Geometry check sheet. Reference: the model listing, model coordinates, mm. A direction names the side the tool comes from. Round coordinates to 2 decimals unless told otherwise and drop trailing zeros. Write each loop counter-clockwise with the first axis right and the second up, starting at its lowest first coordinate (ties: lowest second). Pieces come first, ordered by that corner, then holes. Notation, with made-up numbers: (-10, 74.5) - (22, 74.5) arc R11 cw to (22, 92.5) - close; hole circle Ø11 at (31.5, 13). An arc over 180 degrees is marked (long way). Return JSON: item names as keys, results as strings.
```python
from build123d import *

# Parameters (mm, degrees)
SKETCH_1_R      = 3.9
EXTRUDE_1_DEPTH = 20
SKETCH_2_R      = 5.636785761
SKETCH_2_R_2    = 2.651196968
EXTRUDE_2_DEPTH = 20


with BuildPart() as part:
    # 스케치1 → 보스-돌출1 (new body)
    with BuildSketch(Plane.XY):
        Circle(SKETCH_1_R)
    extrude(amount=EXTRUDE_1_DEPTH)

    # 스케치2 → 보스-돌출2 (add)
    with BuildSketch(Plane.XY):
        Circle(SKETCH_2_R)
        Circle(SKETCH_2_R_2, mode=Mode.SUBTRACT)
    extrude(amount=-EXTRUDE_2_DEPTH)


solid = part.part
```
(1) Section check D-D, the plane y = 3. Enter the section's corners in (x, z), plus the area to 3 significant figures.
Response values:
{"outline": "(-4.77, -20) - (4.77, -20) - (4.77, 0) - (2.49, 0) - (2.49, 20) - (-2.49, 20) - (-2.49, 0) - (-4.77, 0) - close", "area": "291 mm^2"}
(2) Material ranges on line 1 along Y through (x, z) = (0, -9.25); line 2 along Z through (x, y) = (-4, -3.5); line 3 along Z through (x, y) = (1.5, 2), recorded low to high. Write a range as [from, to].
Response values:
{"line 1": "y = [-5.64, -2.65], [2.65, 5.64]", "line 2": "z = [-20, 0]", "line 3": "z = [0, 20]"}
(3) Section check B-B, the plane z = -2. Enter the section's corners in (x, y).
Response values:
{"outline": "circle Ø11.27 at (0, 0); hole circle Ø5.3 at (0, 0)"}
(4) Section check A-A, the plane x = 0. Enter the section's corners in (y, z).
Response values:
{"outline": "(-5.64, -20) - (-2.65, -20) - (-2.65, 0) - (2.65, 0) - (2.65, -20) - (5.64, -20) - (5.64, 0) - (3.9, 0) - (3.9, 20) - (-3.9, 20) - (-3.9, 0) - (-5.64, 0) - close"}
(5) Release check for a two-part mould opening along Y. For faces 4 (the face through (0, 0, 0)), 5 (the face through (-4.155, 3.81, -9.86)), 6 (the face through (1, 3, -20)) record: pulls with the +Y half, pulls with the -Y half, needs draft (parallel to the pull), parting line crosses it, or undercut.
Response values:
{"face 4": "undercut", "face 5": "parting line crosses it", "face 6": "needs draft"}
(6) Gauge pin test, flat ends, axial feed: pin 1 (6 mm diameter, centred on x = 2, z = 8.5, fed in from +Y); pin 2 (6 mm diameter, centred on y = 4, z = 12, fed in from +X); pin 3 (2 mm diameter, centred on x = -4, z = 14.5, fed in from +Y). Record the tip position at first contact, or that the pin passes through.
Response values:
{"pin 1": "stops at y = 3.9", "pin 2": "stops at x = 3.77", "pin 3": "stops at y = 2.49"}
(7) Access from +Z, -Z, +X, -X, +Y, -Y to the whole of each face (thin tool, end or side, straight path). Record for faces 1 (the face through (0, 0, 20)), 2 (the face through (-2.87, 2.64, 9.86)), 3 (the face through (2.529, 0.796, -9.86)).
Response values:
{"face 1": "+Z, +X, -X, +Y, -Y", "face 2": "+Z", "face 3": "-Z"}
